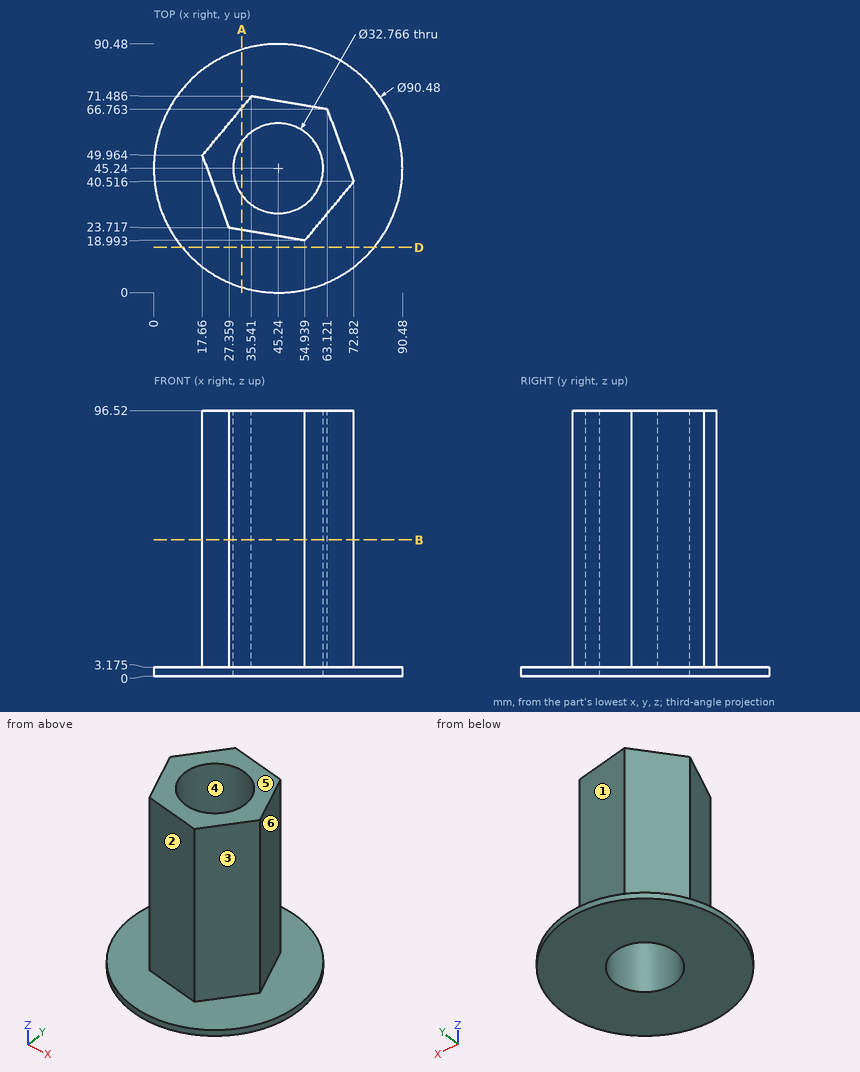
Geometry: see drawing. Coordinates: mm, zero at the bounding-box minimum. A direction names the side the tool comes from. Give positions to 0.01 mm unless a question says otherwise; leave off trailing zeros. Order: outer loops, then holes, each group sorted by start corner. A loop starts at its lowest first (then second) coordinate and runs counter-clockwise, first axis right, second up. Notation, with made-up numbers: M 51,-16.75 L 89,-16.75 A20 ccw 89,13.25 Z; hole C 49.25,41 d7. An arc over 180 degrees is marked long. Answer as CSV lines item,"result". Start each with the question number.
1) Mould query, pull axis Y, two halves, no side actions, for the marked faces 4, 5 and 6. Classes: +Y half, -Y half, draft (parallel to the pull), parting line (faces both ways), or undercut.
2) Cut plane A-A (x = 32). Output: boundary loops of the cut face in (y, z) (1 decimal).
3) Cut plane B-B (z = 49.5). Output: boundary loops of the cut face in (x, y), then the cut area to 3 significant figures.
4) Line query: line 1 (Z direction, x = 13, y = 37) (1 decimal); line 2 (Y direction, x = 37.5, z = 6); line 3 (Y direction, x = 51, z = 9). Output: solid intervals per line, ascending. Write a range as from..to.
5) Cut plane D-D (y = 16.5). Output: boundary loops of the cut face in (x, z) (1 decimal), then the cut area to 3 significant figures.
6) First-contact query: P1, Ø6, axis at x = 53, y = 76.5, coming from the +Z side (3 decimals); P2, Ø1, axis at x = 22.5, y = 50.5, coming from the -Z side; P3, Ø8, axis at y = 31, z = 61, coming from the -X side; P4, Ø8, axis at y = 40.5, z = 52.5, coming from the -X side. Flat tips, straight axial feed; report the tip coordinate or a pass-through.
7) Set-up query: the marked faces 1, 2 and 3. Return all of +Z, -Z, +X, -X, +Y, -Y with unobstructed straight access to the full face (end or side cutting, diameter ignored); none if empty.
Findings below:
1,face 4,"undercut"
1,face 5,"draft"
1,face 6,"+Y half"
2,outline,"M 2,0 L 35.6,0 L 35.6,96.5 L 22.9,96.5 L 22.9,3.2 L 2,3.2 Z; M 54.9,0 L 88.5,0 L 88.5,3.2 L 67.2,3.2 L 67.2,96.5 L 54.9,96.5 Z"
3,outline,"M 17.66,49.96 L 27.36,23.72 L 54.94,18.99 L 72.82,40.52 L 63.12,66.76 L 35.54,71.49 Z; hole C 45.24,45.24 d32.77"
3,area,"1,190 mm²"
4,line 1,"z = 0..3.2"
4,line 2,"y = 21.98..30.8, 59.68..71.15"
4,line 3,"y = 19.67..29.9, 60.58..68.84"
5,outline,"M 10.3,0 L 80.2,0 L 80.2,3.2 L 10.3,3.2 Z"
5,area,"222 mm²"
6,P1,"stops at z = 3.175"
6,P2,"stops at z = 0"
6,P3,"stops at x = 23.19"
6,P4,"stops at x = 19.68"
7,face 1,"+Z, +X, +Y"
7,face 2,"+Z, -X, -Y"
7,face 3,"+Z, +X, -Y"
